Read the model definition and answer for the solid it produces. Units are mm, in the model's axes. Face numbers are marked on the shaded views. Give positions to 0.01 mm unless a question says otherwise; leave off trailing zeros. Write each loop counter-clockwise with the first axis right and the second up, starting at its lowest first coordinate (ties: lowest second). Pieces come first, ordered by that corner, then holes. Notation, with made-up numbers: (85, 63.25) -> (103, 63.25) arc R11 cw to (103, 84.25) -> close; hole circle Ø11 at (-5, 27). An arc over 180 degrees is marked (long way). Use a Markdown table: item, result.
from build123d import *

# Parameters (mm, degrees)
ESQUISSE1_R             = 15
BOSS_EXTRU_1_DEPTH      = 2
ESQUISSE2_R             = 1.5
ENL_V_MAT_EXTRU_1_DEPTH = 3
ESQUISSE3_R             = 1.5
ENL_V_MAT_EXTRU_2_DEPTH = 3
BOSS_EXTRU_2_START      = -4
ESQUISSE4_R             = 3
ESQUISSE4_R_2           = 1.5
BOSS_EXTRU_2_DEPTH      = 4


with BuildPart() as part:
    # Esquisse1 → Boss.-Extru.1 (new body)
    with BuildSketch(Plane.XY):
        Circle(ESQUISSE1_R)
    extrude(amount=BOSS_EXTRU_1_DEPTH)

    # Esquisse2 → Enlèv. mat.-Extru.1 (cut)
    with BuildSketch(Plane.XY.offset(2)):
        Circle(ESQUISSE2_R)
    extrude(amount=-ENL_V_MAT_EXTRU_1_DEPTH, mode=Mode.SUBTRACT)

    # Esquisse3 → Enlèv. mat.-Extru.2 (cut)
    with BuildSketch(Plane.XY.offset(2)):
        with Locations((0, -12)):
            Circle(ESQUISSE3_R)
    extrude(amount=-ENL_V_MAT_EXTRU_2_DEPTH, mode=Mode.SUBTRACT)

    # Esquisse4 → Boss.-Extru.2 (add)
    with BuildSketch(Plane(origin=(0, 0, 0), x_dir=(-1, 0, 0), z_dir=(0, 0, -1)).offset(BOSS_EXTRU_2_START)):
        with Locations((0, -12)):
            Circle(ESQUISSE4_R)
        with Locations(Location((0, -12, 0), (0, 0, 180))):
            Circle(ESQUISSE4_R_2, mode=Mode.SUBTRACT)
    extrude(amount=BOSS_EXTRU_2_DEPTH)


solid = part.part
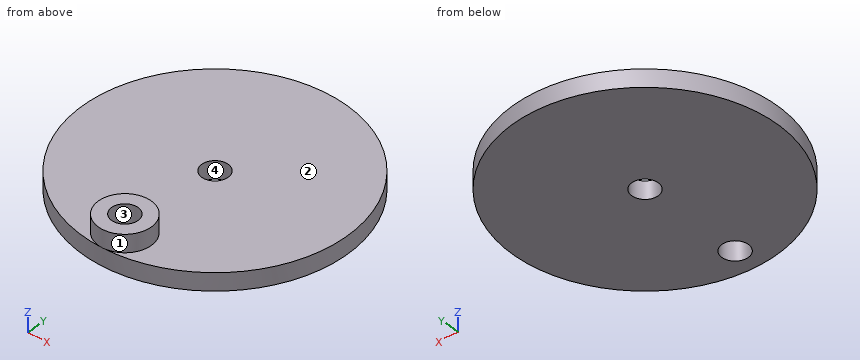
Item 1: A cutting plane is placed at C-C (y = -12). Give the vertices of the cut face in (x, z).
Return value:
| item | result |
|---|---|
| outline | (-9, 0) -> (-1.5, 0) -> (-1.5, 4) -> (-3, 4) -> (-3, 2) -> (-9, 2) -> close; (1.5, 0) -> (9, 0) -> (9, 2) -> (3, 2) -> (3, 4) -> (1.5, 4) -> close |
Item 2: A cutting plane is placed at D-D (z = 2.8). Give the vertices of the cut face in (x, y), then the cut area to 3 significant figures.
Return value:
| item | result |
|---|---|
| outline | circle Ø6 at (0, -12); hole circle Ø3 at (0, -12) |
| area | 21.2 mm^2 |
Item 3: Straight lines are drawn through the part: line 1 along Y through (x, z) = (0, 1.3); line 2 along X through (y, z) = (-12, 2.5); line 3 along Y through (x, z) = (0, 2.35). For each, find the intervals that lie inside material, in ascending order. Write a range as [from, to].
Return value:
| item | result |
|---|---|
| line 1 | [-15, -13.5], [-10.5, -1.5], [1.5, 15] |
| line 2 | [-3, -1.5], [1.5, 3] |
| line 3 | [-15, -13.5], [-10.5, -9] |
Item 4: A cutting plane is placed at A-A (y = 0). Give the vertices of the cut face in (x, z), then the cut area to 3 significant figures.
Return value:
| item | result |
|---|---|
| outline | (-15, 0) -> (-1.5, 0) -> (-1.5, 2) -> (-15, 2) -> close; (1.5, 0) -> (15, 0) -> (15, 2) -> (1.5, 2) -> close |
| area | 54.0 mm^2 |
Item 5: For a pull along X with two mould halves and no side action, classify the marked faces 1, 2, 3 and 4 as +X half, -X half, draft (parallel to the pull), parting line (faces both ways), or undercut.
Return value:
| item | result |
|---|---|
| face 1 | parting line |
| face 2 | draft |
| face 3 | undercut |
| face 4 | undercut |
Item 6: Each of these flat-tipped pins is pushed along its axis until it touches: P1, Ø10, axis at x = 11, y = -2, coming from the +Z side; P2, Ø2, axis at y = 10, z = 2, coming from the +X side; P3, Ø2.5, axis at x = 0, y = 0, coming from the -Z side. Where does it stop, or does it pass through?
Return value:
| item | result |
|---|---|
| P1 | z = 2 |
| P2 | x = 12 |
| P3 | through |
Item 7: A cutting plane is placed at B-B (z = 0.45). Give the vertices of the cut face in (x, y), then the cut area to 3 significant figures.
Return value:
| item | result |
|---|---|
| outline | circle Ø30 at (0, 0); hole circle Ø3 at (0, -12); hole circle Ø3 at (0, 0) |
| area | 693 mm^2 |
